```python
from build123d import *

# Parameters (mm, degrees)
SKETCH1_W               = 29.520850198
SKETCH1_H               = 50.018346185
BOSS_EXTRUDE1_DEPTH     = 10
CUT_EXTRUDE1_DEPTH      = 59.934841575
CUT_EXTRUDE1_DEPTH_BACK = 59.934841575
SKETCH2_R               = 7.812618591


with BuildPart() as part:
    # Sketch1 → Boss-Extrude1 (new body)
    with BuildSketch(Plane(origin=(0, 0, 0), x_dir=(1, 0, 0), z_dir=(0, 1, 0))):
        with Locations((14.760425099, 25.009173093)):
            Rectangle(SKETCH1_W, SKETCH1_H)
    extrude(amount=BOSS_EXTRUDE1_DEPTH)

    # Sketch2 → Cut-Extrude1 (cut, two sides: drawn at the far end of the back side and taken through both)
    with BuildSketch(Plane(origin=(0, 10, 0), x_dir=(1, 0, 0), z_dir=(0, 1, 0)).offset(-CUT_EXTRUDE1_DEPTH_BACK)):
        with Locations(Location((14.760425099, 26.187461577, 0), (0, 0, 270))):
            Circle(SKETCH2_R)
    extrude(amount=CUT_EXTRUDE1_DEPTH + CUT_EXTRUDE1_DEPTH_BACK, mode=Mode.SUBTRACT)


solid = part.part
```
The model under review builds one solid part; all positions refer to its coordinate system, in mm. Coordinates: 2 decimals unless noted, no trailing zeros. Write each loop counter-clockwise with the first axis right and the second up, starting at its lowest first coordinate (ties: lowest second). Pieces come first, ordered by that corner, then holes.
1) Clearance check with a flat-ended pin moving along its axis: pin 1 Ø14 at (x, z) = (14.76, -26.19) entering from +Y (3 decimals). State where the tip first meets the part, or that it passes through.
2) We need section A-A on z = -27. State the section outline as (x, y) points, then the cut area to 3 significant figures.
3) We need section C-C on y = 8. State the section outline as (x, z) points, then the cut area to 3 significant figures.
4) To check wall thickness, follow probe 1 along X at (y, z) = (8.5, -30); probe 2 along X at (y, z) = (4.5, -19); probe 3 along Z at (x, y) = (12.5, 5). State the ranges of each line that lie inside material, in increasing order.
5) The part is to be moulded in two halves that separate along X. For faces 1 (the face through (29.521, 5, -25)), 2 (the face through (21, 0, -20)), 3 (the face through (11.77, 4.93, -18.97)), say which applies: pulls with the +X half, pulls with the -X half, needs draft (parallel to the pull), parting line crosses it, or undercut.
6) We need section B-B on x = 20.25. State the section outline as (y, z) points.
Answer list:
1. pin 1: passes through
2. outline: (0, 0) - (6.99, 0) - (6.99, 10) - (0, 10) - close; (22.53, 0) - (29.52, 0) - (29.52, 10) - (22.53, 10) - close
2. area: 140 mm2
3. outline: (0, -50.02) - (29.52, -50.02) - (29.52, 0) - (0, 0) - close; hole circle Ø15.63 at (14.76, -26.19)
3. area: 1,280 mm2
4. probe 1: x = 0 to 7.94, 21.58 to 29.52
4. probe 2: x = 0 to 11.7, 17.82 to 29.52
4. probe 3: z = -50.02 to -33.67, -18.71 to 0
5. face 1: pulls with the +X half
5. face 2: needs draft
5. face 3: undercut
6. outline: (0, -50.02) - (10, -50.02) - (10, -31.75) - (0, -31.75) - close; (0, -20.63) - (10, -20.63) - (10, 0) - (0, 0) - close
